```python
from build123d import *

# Parameters (mm, degrees)
BOSS_EXTRUDE1_DEPTH = 40
SKETCH2_R           = 1.5
CUT_EXTRUDE1_DEPTH  = 10


with BuildPart() as part:
    # Sketch1 → Boss-Extrude1 (new body)
    with BuildSketch(Plane(origin=(0, 0, 0), x_dir=(1, 0, 0), z_dir=(0, 1, 0))):
        Polygon((3.175426481, 0), (1.58771324, 2.75), (-1.58771324, 2.75), (-3.175426481, 0), (-1.58771324, -2.75), (1.58771324, -2.75), align=None)
    extrude(amount=BOSS_EXTRUDE1_DEPTH)

    # Sketch2 → Cut-Extrude1 (cut)
    with BuildSketch(Plane(origin=(0, 40, 0), x_dir=(1, 0, 0), z_dir=(0, 1, 0))):
        Circle(SKETCH2_R)
    cut_extrude1 = extrude(amount=-CUT_EXTRUDE1_DEPTH, mode=Mode.SUBTRACT)

    # Mirror1: Cut-Extrude1 across plane
    add(cut_extrude1.mirror(Plane(origin=(0, 20, 0), x_dir=(0, 0, 1), z_dir=(0, -1, 0))), mode=Mode.SUBTRACT)


solid = part.part
```
The model under review builds one solid part; all positions refer to its coordinate system, in mm. A direction names the side the tool comes from. Give positions to 0.01 mm unless a question says otherwise; leave off trailing zeros. Loops run counter-clockwise (first coordinate to the right, second up) from the corner with the lowest first, then second, coordinate; pieces in that order, holes last. Notation, with made-up numbers: (39.25, 3) - (60.25, 3) arc R22 ccw to (60.25, 41) - close; hole circle Ø2 at (-38.75, 74). An arc over 180 degrees is marked (long way). Answer as a JSON object with one key per item and string values.
Q1. Insertion check: pin 1 (1.5 mm diameter, centred on x = 0.5, z = 0.5, fed in from +Y); pin 2 (1.5 mm diameter, centred on x = -0.5, z = -1, fed in from +Y); pin 3 (2.5 mm diameter, centred on x = 0, z = 0, fed in from -Y). Each pin has a flat end and moves straight along its axis. Give the tip position at first contact, or say it passes through.
Worked out:
{"pin 1": "stops at y = 30", "pin 2": "stops at y = 40", "pin 3": "stops at y = 10"}
Q2. Add section D-D on y = 22.5. State the section outline as (x, z) points.
Worked out:
{"outline": "(-3.18, 0) - (-1.59, -2.75) - (1.59, -2.75) - (3.18, 0) - (1.59, 2.75) - (-1.59, 2.75) - close"}
Q3. Add section A-A on y = 35. State the section outline as (x, z) points.
Worked out:
{"outline": "(-3.18, 0) - (-1.59, -2.75) - (1.59, -2.75) - (3.18, 0) - (1.59, 2.75) - (-1.59, 2.75) - close; hole circle Ø3 at (0, 0)"}
Q4. To check wall thickness, follow line 1 along Z through (x, y) = (0, 3.5); line 2 along X through (y, z) = (3, 0.95); line 3 along Z through (x, y) = (-1, 4). State the ranges of each line that lie inside material, in increasing order.
Worked out:
{"line 1": "z = -2.75 to -1.5, 1.5 to 2.75", "line 2": "x = -2.63 to -1.16, 1.16 to 2.63", "line 3": "z = -2.75 to -1.12, 1.12 to 2.75"}
Q5. Add section C-C on z = -0.55. State the section outline as (x, y) points.
Worked out:
{"outline": "(-2.86, 0) - (-1.4, 0) - (-1.4, 10) - (1.4, 10) - (1.4, 0) - (2.86, 0) - (2.86, 40) - (1.4, 40) - (1.4, 30) - (-1.4, 30) - (-1.4, 40) - (-2.86, 40) - close"}
Q6. For faces 1 (the flat face through (0, 30, 0)), 2 (the flat face through (0, 20, -2.75)), 3 (the cylindrical face through (-1.5, 4.93, -0.07)), list the 3-axis set-ups (+Z, -Z, +X, -X, +Y, -Y) from which the entire face can be reached by the end or side of a thin tool; tool diameter is ignored.
Worked out:
{"face 1": "+Y", "face 2": "-Z, +X, -X, +Y, -Y", "face 3": "-Y"}
Q7. Add section B-B on x = 0. State the section outline as (y, z) points.
Worked out:
{"outline": "(0, -2.75) - (40, -2.75) - (40, -1.5) - (30, -1.5) - (30, 1.5) - (40, 1.5) - (40, 2.75) - (0, 2.75) - (0, 1.5) - (10, 1.5) - (10, -1.5) - (0, -1.5) - close"}
